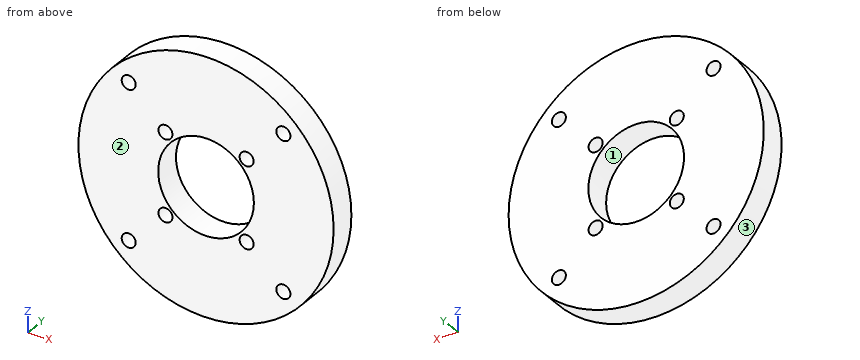
```python
from build123d import *

# Parameters (mm, degrees)
F0_R     = 20
F0_R_2   = 1.1
F0_R_3   = 7.5
F1_DEPTH = 4.318


with BuildPart() as f1:
    # F0 (on Front) → F1 (new body)
    with BuildSketch(Plane.XZ):
        Circle(F0_R)
        with Locations((-12.123346, -12.123346)):
            Circle(F0_R_2, mode=Mode.SUBTRACT)
        with Locations((-6.363961, -6.363961)):
            Circle(F0_R_2, mode=Mode.SUBTRACT)
        with Locations((12.123346, -12.123346)):
            Circle(F0_R_2, mode=Mode.SUBTRACT)
        with Locations((6.363961, -6.363961)):
            Circle(F0_R_2, mode=Mode.SUBTRACT)
        with Locations((-6.363961, 6.363961)):
            Circle(F0_R_2, mode=Mode.SUBTRACT)
        with Locations((-12.123346, 12.123346)):
            Circle(F0_R_2, mode=Mode.SUBTRACT)
        Circle(F0_R_3, mode=Mode.SUBTRACT)
        with Locations((6.363961, 6.363961)):
            Circle(F0_R_2, mode=Mode.SUBTRACT)
        with Locations((12.123346, 12.123346)):
            Circle(F0_R_2, mode=Mode.SUBTRACT)
    extrude(amount=F1_DEPTH)


solid = f1.part
```
Could you check a few things on this model? Use its own coordinates, in mm. Face numbers are marked on the shaded views. Round coordinates to 2 decimals unless told otherwise and drop trailing zeros. Loops run counter-clockwise (first coordinate to the right, second up) from the corner with the lowest first, then second, coordinate; pieces in that order, holes last. Notation, with made-up numbers: (59, 10.25) - (67, 10.25) arc R35 cw to (67, 48.25) - close; hole circle Ø11 at (6, -23). An arc over 180 degrees is marked (long way). Use CSV: the item, a comma, the result in double quotes.
Item 1: If we section it at A-A on z = 0: List the corners of the cut face in (x, y) for me, then the cut area to 3 significant figures.
Here are the results:
outline,"(-20, -4.32) - (-7.5, -4.32) - (-7.5, 0) - (-20, 0) - close; (7.5, -4.32) - (20, -4.32) - (20, 0) - (7.5, 0) - close"
area,"108 mm²"
Item 2: I need wall thicknesses on L1, parallel to Z at x = -5.5, y = -3.55; L2, parallel to Z at x = -12.5, y = -0.65; L3, parallel to Z at x = -15, y = -1.8. Which ranges of each line are inside material? Lowest first, please. Write a range as [from, to].
Here are the results:
L1,"z = [-19.23, -7.04], [-5.68, -5.1], [5.1, 5.68], [7.04, 19.23]"
L2,"z = [-15.61, -13.16], [-11.09, 11.09], [13.16, 15.61]"
L3,"z = [-13.23, 13.23]"
Item 3: If we mould it in two halves opening along X, with no side actions, what happens to the marked faces 1, 2 and 3? For each: pulls with the +X half, pulls with the -X half, needs draft (parallel to the pull), parting line crosses it, or undercut.
Here are the results:
face 1,"undercut"
face 2,"needs draft"
face 3,"parting line crosses it"
Item 4: If we section it at B-B on x = 0: List the corners of the cut face in (y, z) for me.
Here are the results:
outline,"(-4.32, -20) - (0, -20) - (0, -7.5) - (-4.32, -7.5) - close; (-4.32, 7.5) - (0, 7.5) - (0, 20) - (-4.32, 20) - close"
Item 5: Will these pins go through, and if not, where does the flat tip stop? pin 1 (2 mm diameter, centred on x = 12.12, z = 12.12, fed in from +Y); pin 2 (2 mm diameter, centred on y = -3, z = -1.5, fed in from +X); pin 3 (2 mm diameter, centred on y = -2, z = 15, fed in from +X); pin 4 (1 mm diameter, centred on y = -3.5, z = 9, fed in from +X).
Here are the results:
pin 1,"passes through"
pin 2,"stops at x = 19.99"
pin 3,"stops at x = 14.28"
pin 4,"stops at x = 18.1"
Item 6: If we section it at D-D on x = -6.5: List the corners of the cut face in (y, z) for me, then the cut area to 3 significant figures.
Here are the results:
outline,"(-4.32, -18.91) - (0, -18.91) - (0, -7.46) - (-4.32, -7.46) - close; (-4.32, -5.27) - (0, -5.27) - (0, -3.74) - (-4.32, -3.74) - close; (-4.32, 3.74) - (0, 3.74) - (0, 5.27) - (-4.32, 5.27) - close; (-4.32, 7.46) - (0, 7.46) - (0, 18.91) - (-4.32, 18.91) - close"
area,"112 mm²"
Item 7: If we section it at C-C on y = -2.8: Count the separate pieces of the cut face and the enclosed holes in it, then the cut area to 3 significant figures.
Here are the results:
separate pieces,"1"
enclosed holes,"9"
area,"1,050 mm²"
